from build123d import *

# Parameters (mm, degrees)
SKETCH_1_W          = 10
SKETCH_1_H          = 10
SKETCH_1_W_2        = 8
SKETCH_1_H_2        = 8
EXTRUDE_1_DEPTH     = 100
SKETCH_2_R          = 2.1
CUT_EXTRUDE_1_DEPTH = 101.623058987
SKETCH_3_R          = 1.6
CUT_EXTRUDE_2_DEPTH = 101.623058987


with BuildPart() as part:
    # ｽｹｯﾁ1 → 押し出し-薄板1 (new body)
    with BuildSketch(Plane(origin=(0, 0, 0), x_dir=(1, 0, 0), z_dir=(0, 1, 0))):
        Rectangle(SKETCH_1_W, SKETCH_1_H)
        Rectangle(SKETCH_1_W_2, SKETCH_1_H_2, mode=Mode.SUBTRACT)
    extrude(amount=EXTRUDE_1_DEPTH)

    # ｽｹｯﾁ2 → ｶｯﾄ - 押し出し1 (cut, through all)
    with BuildSketch(Plane(origin=(5, 0, 0), x_dir=(0, 0, -1), z_dir=(1, 0, 0))):
        with Locations((0, 5)):
            Circle(SKETCH_2_R)
    extrude(amount=-CUT_EXTRUDE_1_DEPTH, mode=Mode.SUBTRACT)

    # ｽｹｯﾁ3 → ｶｯﾄ - 押し出し2 (cut, through all)
    with BuildSketch(Plane.XY.offset(5)):
        with Locations((0, 85)):
            Circle(SKETCH_3_R)
        with Locations((0, 95)):
            Circle(SKETCH_3_R)
    extrude(amount=-CUT_EXTRUDE_2_DEPTH, mode=Mode.SUBTRACT)


solid = part.part
Work out the finished part from the listing and answer in its coordinate system (mm). A direction names the side the tool comes from. Give positions to 0.01 mm unless a question says otherwise; leave off trailing zeros. Order: outer loops, then holes, each group sorted by start corner. A loop starts at its lowest first (then second) coordinate and runs counter-clockwise, first axis right, second up. Notation, with made-up numbers: (40, 52) -> (46, 52) arc R21 ccw to (46, 71) -> close; hole circle Ø11 at (4.25, 81.5). An arc over 180 degrees is marked (long way). One line per item, written item: value.
Item 1: A tool of negligible diameter and unlimited length cuts with its end or side. For faces 1 (the flat face through (-4, 49, 0)), 2 (the cylindrical face through (4.507, 7.082, 0.273)), from which of +Z, -Z, +X, -X, +Y, -Y can it reach the whole face along a straight path? Write none if from no direction.
Answer sheet:
face 1: +Y, -Y
face 2: +X, -X
Item 2: A flat-ended cylindrical pin translates along its axis: P1, Ø1.9, axis at x = 0, y = 95, coming from the +Z side. Find the tip coordinate at first contact, or state that the pin passes through.
Answer sheet:
P1: through
Item 3: Straight lines are drawn through the part: probe 1 along Y at (x, z) = (0, -4.5); probe 2 along X at (y, z) = (55, -3.25). For each, find the intervals that lie inside material, in ascending order.
Answer sheet:
probe 1: 0 to 83.4, 86.6 to 93.4, 96.6 to 100
probe 2: -5 to -4, 4 to 5
Item 4: Determine the mould class of faces 3 (the cylindrical face through (-0.208, 96.586, -4.493)), 4 (the flat face through (0, 49, -5)), 5 (the flat face through (0, 49, 4)) for opening direction Z: released by +Z, released by -Z, zero draft, split by the parting line, or undercut.
Answer sheet:
face 3: zero draft
face 4: released by -Z
face 5: undercut
Item 5: Find section B-B, the plane z = 0. Give the vertices of the cut face in (x, y), plus the area to 3 significant figures.
Answer sheet:
outline: (-5, 0) -> (-4, 0) -> (-4, 2.9) -> (-5, 2.9) -> close; (-5, 7.1) -> (-4, 7.1) -> (-4, 100) -> (-5, 100) -> close; (4, 0) -> (5, 0) -> (5, 2.9) -> (4, 2.9) -> close; (4, 7.1) -> (5, 7.1) -> (5, 100) -> (4, 100) -> close
area: 192 mm²
Item 6: Find section A-A, the plane y = 5. Give the vertices of the cut face in (x, z), plus the area to 3 significant figures.
Answer sheet:
outline: (-5, -5) -> (5, -5) -> (5, -2.1) -> (4, -2.1) -> (4, -4) -> (-4, -4) -> (-4, -2.1) -> (-5, -2.1) -> close; (-5, 2.1) -> (-4, 2.1) -> (-4, 4) -> (4, 4) -> (4, 2.1) -> (5, 2.1) -> (5, 5) -> (-5, 5) -> close
area: 27.6 mm²
Item 7: Find section C-C, the plane x = -0.5. Give the vertices of the cut face in (y, z).
Answer sheet:
outline: (0, -5) -> (83.48, -5) -> (83.48, -4) -> (0, -4) -> close; (0, 4) -> (83.48, 4) -> (83.48, 5) -> (0, 5) -> close; (86.52, -5) -> (93.48, -5) -> (93.48, -4) -> (86.52, -4) -> close; (86.52, 4) -> (93.48, 4) -> (93.48, 5) -> (86.52, 5) -> close; (96.52, -5) -> (100, -5) -> (100, -4) -> (96.52, -4) -> close; (96.52, 4) -> (100, 4) -> (100, 5) -> (96.52, 5) -> close
Item 8: Find section D-D, the plane y = 79. Give the vertices of the cut face in (x, z), plus the area to 3 significant figures.
Answer sheet:
outline: (-5, -5) -> (5, -5) -> (5, 5) -> (-5, 5) -> close; hole (-4, -4) -> (4, -4) -> (4, 4) -> (-4, 4) -> close
area: 36.0 mm²
